Verification items for the finished model (mm, model axes). Face numbers are marked on the shaded views. Round coordinates to 2 decimals unless told otherwise and drop trailing zeros. Write each loop counter-clockwise with the first axis right and the second up, starting at its lowest first coordinate (ties: lowest second). Pieces come first, ordered by that corner, then holes. Notation, with made-up numbers: (-21.5, 60.5) -> (-13.5, 60.5) arc R21 cw to (-13.5, 75.5) -> close; hole circle Ø9 at (-25.75, 81.5). An arc over 180 degrees is marked (long way). Answer as a JSON object with one key per item and string values. Group by question number.
(1) Gauge pin test, flat end, axial feed: pin 1 Ø15.5 at (y, z) = (-29, 3.5) entering from +X. Record the tip position at first contact, or that the pin passes through.
(2) Sectioned sample at B-B on x = 14. Record the cut outline in (y, z), and give its area (3 significant figures).
(3) Scan lines: L1, parallel to Z at x = 40, y = -25; L2, parallel to Z at x = -38.5, y = -25; L3, parallel to Y at x = -4, z = 6. Record each from-to range of solid material in increasing order. Write a range as from..to.
(4) Sectioned sample at A-A on y = -25. Record the cut outline in (x, z), and give its area (3 significant figures).
(5) Sectioned sample at C-C on z = 2.5. Record the cut outline in (x, y), and give its area (3 significant figures).
(6) Sectioned sample at D-D on x = -13. Record the cut outline in (y, z).
(7) Draft check along Z on the marked faces 1, 2 and 3. Enter one of: released by +Z, released by -Z, zero draft, split by the parting line, or undercut.
```python
from build123d import *

# Parameters (mm, degrees)
F0_W     = 100
F0_H     = 100
F1_DEPTH = 50
F2_R     = 10
F3_SIZE  = 5
F4_R     = 15.391397
F5_DEPTH = 50
F6_R     = 10
F7_DEPTH = 50


with BuildPart() as f1:
    # F0 (on Front) → F1 (new body)
    with BuildSketch(Plane.XZ):
        Rectangle(F0_W, F0_H)
    extrude(amount=F1_DEPTH)

    # F2
    f2_edges = [f1.edges().sort_by_distance(p)[0] for p in [
        (-50, -25, 50),
    ]]
    fillet(f2_edges, radius=F2_R)

    # F3
    f3_edges = [f1.edges().sort_by_distance(p)[0] for p in [
        (50, -25, -50),
    ]]
    chamfer(f3_edges, length=F3_SIZE)

    # F4 (on face) → F5 (cut)
    with BuildSketch(Plane.YZ.offset(50)):
        with Locations((-25, 2.5)):
            Circle(F4_R)
    extrude(amount=-F5_DEPTH, mode=Mode.SUBTRACT)

    # F6 (on face) → F7 (cut)
    with BuildSketch(Plane(origin=(-50, 0, 0), x_dir=(0, -1, 0), z_dir=(-1, 0, 0))):
        with Locations((25, 0)):
            Circle(F6_R)
    extrude(amount=-F7_DEPTH, mode=Mode.SUBTRACT)


solid = f1.part
```
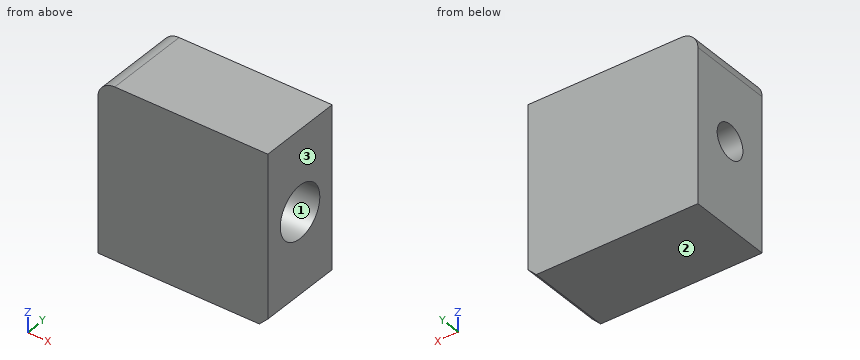
Computed values:
{
 "1": {"pin 1": "x = 0"},
 "2": {"outline": "(-50, -50) -> (0, -50) -> (0, 50) -> (-50, 50) -> close; hole circle Ø30.78 at (-25, 2.5)", "area": "4,260 mm2"},
 "3": {"L1": "-50..-12.89, 17.89..50", "L2": "-50..-10, 10..50", "L3": "-50..-33, -17..0"},
 "4": {"outline": "(-50, -50) -> (45, -50) -> (50, -45) -> (50, -12.89) -> (0, -12.89) -> (0, -10) -> (-50, -10) -> close; (-50, 10) -> (0, 10) -> (0, 17.89) -> (50, 17.89) -> (50, 50) -> (-40, 50) arc R10 ccw to (-50, 40) -> close", "area": "7,430 mm2"},
 "5": {"outline": "(-50, -50) -> (50, -50) -> (50, -40.39) -> (0, -40.39) -> (0, -34.68) -> (-50, -34.68) -> close; (-50, -15.32) -> (0, -15.32) -> (0, -9.61) -> (50, -9.61) -> (50, 0) -> (-50, 0) -> close", "area": "2,490 mm2"},
 "6": {"outline": "(-50, -50) -> (0, -50) -> (0, 50) -> (-50, 50) -> close; hole circle Ø20 at (-25, 0)"},
 "7": {"face 1": "undercut", "face 2": "released by -Z", "face 3": "zero draft"}
}
